```python
from build123d import *

# Parameters (mm, degrees)
SKETCH1_W         = 50.8
SKETCH1_H         = 10.16
SKETCH1_R         = 1.15
PCB_DEPTH         = 1.6
SKETCH2_W         = 4.9
SKETCH2_H         = 4.9
LEDS_DEPTH        = 1.5
SKETCH3_W         = 2
SKETCH3_H         = 1.3
CAPS_DEPTH        = 1.3
SKETCH4_R         = 2
LED_WINDOWS_DEPTH = 0.1
FILED_FILLETS_R   = 1


with BuildPart() as part:
    # Sketch1 → PCB (new body)
    with BuildSketch(Plane(origin=(0, 0, 0), x_dir=(1, 0, 0), z_dir=(0, 1, 0))):
        Rectangle(SKETCH1_W, SKETCH1_H)
        with Locations((-12.7, 3.048)):
            Circle(SKETCH1_R, mode=Mode.SUBTRACT)
        with Locations((12.7, 3.048)):
            Circle(SKETCH1_R, mode=Mode.SUBTRACT)
    extrude(amount=PCB_DEPTH)

    # Sketch2 → LEDs (add)
    with BuildSketch(Plane(origin=(0, 1.6, 0), x_dir=(1, 0, 0), z_dir=(0, 1, 0))):
        with Locations((3.175, -1.28)):
            Rectangle(SKETCH2_W, SKETCH2_H)
        with Locations((-3.175, -1.28)):
            Rectangle(SKETCH2_W, SKETCH2_H)
        with Locations((9.525, -1.28)):
            Rectangle(SKETCH2_W, SKETCH2_H)
        with Locations((15.875, -1.28)):
            Rectangle(SKETCH2_W, SKETCH2_H)
        with Locations((22.225, -1.28)):
            Rectangle(SKETCH2_W, SKETCH2_H)
        with Locations((-22.225, -1.28)):
            Rectangle(SKETCH2_W, SKETCH2_H)
        with Locations((-15.875, -1.28)):
            Rectangle(SKETCH2_W, SKETCH2_H)
        with Locations((-9.525, -1.28)):
            Rectangle(SKETCH2_W, SKETCH2_H)
    extrude(amount=LEDS_DEPTH)

    # Sketch3 → Caps (add)
    with BuildSketch(Plane(origin=(0, 1.6, 0), x_dir=(1, 0, 0), z_dir=(0, 1, 0))):
        with Locations((-15.875, 3.048)):
            Rectangle(SKETCH3_W, SKETCH3_H)
        with Locations((-22.225, 3.048)):
            Rectangle(SKETCH3_W, SKETCH3_H)
        with Locations((-9.525, 3.048)):
            Rectangle(SKETCH3_W, SKETCH3_H)
        with Locations((-3.175, 3.048)):
            Rectangle(SKETCH3_W, SKETCH3_H)
        with Locations((3.175, 3.048)):
            Rectangle(SKETCH3_W, SKETCH3_H)
        with Locations((9.525, 3.048)):
            Rectangle(SKETCH3_W, SKETCH3_H)
        with Locations((15.875, 3.048)):
            Rectangle(SKETCH3_W, SKETCH3_H)
        with Locations((22.225, 3.048)):
            Rectangle(SKETCH3_W, SKETCH3_H)
    extrude(amount=CAPS_DEPTH)

    # Sketch4 → LED windows (cut)
    with BuildSketch(Plane(origin=(0, 3.1, 0), x_dir=(1, 0, 0), z_dir=(0, 1, 0))):
        with Locations((-22.225, -1.28)):
            Circle(SKETCH4_R)
        with Locations((-15.875, -1.28)):
            Circle(SKETCH4_R)
        with Locations((-9.525, -1.28)):
            Circle(SKETCH4_R)
        with Locations((-3.175, -1.28)):
            Circle(SKETCH4_R)
        with Locations((3.175, -1.28)):
            Circle(SKETCH4_R)
        with Locations((9.525, -1.28)):
            Circle(SKETCH4_R)
        with Locations((15.875, -1.28)):
            Circle(SKETCH4_R)
        with Locations((22.225, -1.28)):
            Circle(SKETCH4_R)
    extrude(amount=-LED_WINDOWS_DEPTH, mode=Mode.SUBTRACT)

    # Filed fillets
    filed_fillets_edges = [part.edges().sort_by_distance(p)[0] for p in [
        (25.4, 0.8, 5.08),
        (-25.4, 0.8, 5.08),
        (-25.4, 0.8, -5.08),
        (25.4, 0.8, -5.08),
    ]]
    fillet(filed_fillets_edges, radius=FILED_FILLETS_R)


solid = part.part
```
The listing builds one solid part. Answer for the finished solid, in the listing's coordinates (mm). A direction names the side the tool comes from. Coordinates: 2 decimals unless noted, no trailing zeros. Write each loop counter-clockwise with the first axis right and the second up, starting at its lowest first coordinate (ties: lowest second). Pieces come first, ordered by that corner, then holes. Notation, with made-up numbers: (-39.75, 3) -> (-35.75, 3) arc R26 cw to (-35.75, 21) -> close; hole circle Ø3 at (32.5, 9). An arc over 180 degrees is marked (long way). Write each question's results on one line, items separated by ' | '. Start each with the question number.
1) For a pull along X with two mould halves and no side action, classify faces 5 (the flat face through (-25.4, 1, 0)), 6 (the flat face through (-8.525, 2, -3)), 7 (the flat face through (0, 1, -5.08)) as +X half, -X half, draft (parallel to the pull), parting line (faces both ways), or undercut.
2) A cutting plane is placed at A-A (x = 12.7). Determine the outline of the cut face in (y, z).
3) A tool of negligible diameter and unlimited length cuts with its end or side. For faces 1 (the flat face through (-10, 2, -2.398)), 2 (the flat face through (-16, 2, 3.73)), 3 (the flat face through (-10, 3, 1)), 4 (the flat face through (2.175, 2, -3)), from which of +Z, -Z, +X, -X, +Y, -Y can it reach the whole face along a straight path? Write none if from no direction.
4) Flat-ended cylindrical pins translate along their axes: pin 1 Ø1.4 at (y, z) = (2, -3) entering from +X; pin 2 Ø0.6 at (y, z) = (2, -3) entering from +X (3 decimals); pin 3 Ø0.8 at (x, y) = (10, 2.5) entering from +Z; pin 4 Ø1.6 at (y, z) = (2.5, 2) entering from -X (3 decimals). Find the tip coordinate at first contact, or state that the pin passes through.
5) Straight lines are drawn through the part: probe 1 along Z at (x, y) = (12.7, 1.1); probe 2 along Y at (x, z) = (-22, -1.75); probe 3 along Y at (x, z) = (2, 0.75). For each, find the intervals that lie inside material, in ascending order.
6) A cutting plane is placed at B-B (y = 0.55). Determine the outline of the cut face in (x, z), then the cut area to 3 significant figures.
7) A cutting plane is placed at C-C (x = -3.5). Determine the outline of the cut face in (y, z).
Values follow:
1) face 5: -X half | face 6: undercut | face 7: draft
2) outline: (0, -5.08) -> (1.6, -5.08) -> (1.6, -4.2) -> (0, -4.2) -> close; (0, -1.9) -> (1.6, -1.9) -> (1.6, 5.08) -> (0, 5.08) -> close
3) face 1: +X, -X, +Y | face 2: +Z, +X, -X, +Y | face 3: +Y | face 4: -Z, +Y
4) pin 1: x = 25.4 | pin 2: x = 23.225 | pin 3: z = 3.73 | pin 4: x = -24.675
5) probe 1: -5.08 to -4.2, -1.9 to 5.08 | probe 2: 0 to 1.6 | probe 3: 0 to 3
6) outline: (-25.4, -4.08) arc R1 ccw to (-24.4, -5.08) -> (24.4, -5.08) arc R1 ccw to (25.4, -4.08) -> (25.4, 4.08) arc R1 ccw to (24.4, 5.08) -> (-24.4, 5.08) arc R1 ccw to (-25.4, 4.08) -> close; hole circle Ø2.3 at (-12.7, -3.05); hole circle Ø2.3 at (12.7, -3.05) | area: 507 mm²
7) outline: (0, -5.08) -> (1.6, -5.08) -> (1.6, -3.7) -> (2.9, -3.7) -> (2.9, -2.4) -> (1.6, -2.4) -> (1.6, -1.17) -> (3.1, -1.17) -> (3.1, -0.69) -> (3, -0.69) -> (3, 3.25) -> (3.1, 3.25) -> (3.1, 3.73) -> (1.6, 3.73) -> (1.6, 5.08) -> (0, 5.08) -> close
